Autodesk Inventor part; units mm, degrees
ref_plane "YZ Plane" through (0, 0, 0) normal (1, 0, 0) x (0, 1, 0)
ref_plane "XZ Plane" through (0, 0, 0) normal (0, 1, 0) x (-1, 0, 0)
ref_plane "XY Plane" through (0, 0, 0) normal (0, 0, 1) x (1, 0, 0)
sketch "Sketch13" plane through (0, 0, 0) normal (0, 0, 1) x (1, 0, 0)
  line L0 (-43, -40) -> (-43, 40)
  circle A0 centre (-35, 32) radius 2.75
  circle A1 centre (-35, -32) radius 2.75
  line L1 (-43, 40) -> (43, 40)
  line L2 (43, 40) -> (43, -40)
  line L3 (43, -40) -> (-43, -40)
  line L4 (0, 40) -> (0, -40) construction
  line L5 (-20, 40) -> (-20, -40) construction
  line L6 (20, 40) -> (20, -40) construction
  line L7 (-43, 0) -> (43, 0) construction
  circle A2 centre (35, 32) radius 2.75
  circle A3 centre (35, -32) radius 2.75
  line L8 (20, 40) -> (-18, 40)
  line L9 (20, -40) -> (-10, -40)
  point P0 (0, 0)
  point P1 (40, 0)
  point P2 (0, 0)
  dimension "d96" = 80
  dimension "d100" = 5.5
  dimension "d101" = 8
  dimension "d106" = 40
  dimension "d107" = 8
  dimension "d111" = 23
extrude "Plate6" add sketch "Sketch13" along normal blind 2
fillet "Fillet4" radius 2 4 edges at (43, 40, 1) (-43, 40, 1) (-43, -40, 1) (43, -40, 1)
equation "\"d108\" = Thickness"
equation "\"BendRadius\" = Thickness"
equation "\"BendReliefWidth\" = Thickness"
equation "\"BendReliefDepth\" = 0.5 * Thickness"
equation "\"CornerReliefSize\" = 4 * Thickness"
equation "\"MinimumRemnant\" = 2 * Thickness"
equation "\"TransitionRadius\" = BendRadius"
equation "\"JacobiRadiusSize\" = BendRadius"
equation "\"GapSize\" = Thickness"
properties part number "NDM 7.47 bracket floor pillar"
For this review, take the finished solid that the model builds, in its own axes (mm). Round coordinates to 2 decimals unless told otherwise and drop trailing zeros. Order: outer loops, then holes, each group sorted by start corner. A loop starts at its lowest first (then second) coordinate and runs counter-clockwise, first axis right, second up. Notation, with made-up numbers: M 8,38 L 27,38 A32 ccw 27,65 Z; hole C -20,36.5 d6. An arc over 180 degrees is marked long. Use a Markdown table: item, result. Add a question column.
Item 1: Add section B-B, the plane y = -32. Give the boundary of the cut face in (x, z), then the cut area to 3 significant figures.
Item 2: Mouldability with a two-part tool opening along X and no side actions: class faces 1 (the flat face through (-1, 1, 2)), 2 (the cylindrical face through (32.973, 30.141, 0.986)), 3 (the cylindrical face through (-42.43, -39.4, 1.01)), 4 (the cylindrical face through (32.973, -33.859, 0.986)) as released by +X, released by -X, zero draft, split by the parting line, or undercut.
Item 3: Insertion check: pin 1 (6.5 mm diameter, centred on x = 35, y = 32, fed in from -Z). The pin has a flat end and moves straight along its axis. Give the tip position at first contact, or say it passes through.
Item 4: To check wall thickness, follow line 1 along Y through (x, z) = (35, 1.4); line 2 along Y through (x, z) = (36, 0.7); line 3 along X through (y, z) = (-31.5, 1.05). State the ranges of each line that lie inside material, in increasing order.
Item 5: Add section A-A, the plane x = 35. Give the boundary of the cut face in (y, z).
Geometry results:
| question | item | result |
|---|---|---|
| 1 | outline | M -43,0 L -37.75,0 L -37.75,2 L -43,2 Z; M -32.25,0 L 32.25,0 L 32.25,2 L -32.25,2 Z; M 37.75,0 L 43,0 L 43,2 L 37.75,2 Z |
| 1 | area | 150 mm² |
| 2 | face 1 | zero draft |
| 2 | face 2 | undercut |
| 2 | face 3 | released by -X |
| 2 | face 4 | undercut |
| 3 | pin 1 | stops at z = 0 |
| 4 | line 1 | y = -40 to -34.75, -29.25 to 29.25, 34.75 to 40 |
| 4 | line 2 | y = -40 to -34.56, -29.44 to 29.44, 34.56 to 40 |
| 4 | line 3 | x = -43 to -37.7, -32.3 to 32.3, 37.7 to 43 |
| 5 | outline | M -40,0 L -34.75,0 L -34.75,2 L -40,2 Z; M -29.25,0 L 29.25,0 L 29.25,2 L -29.25,2 Z; M 34.75,0 L 40,0 L 40,2 L 34.75,2 Z |
